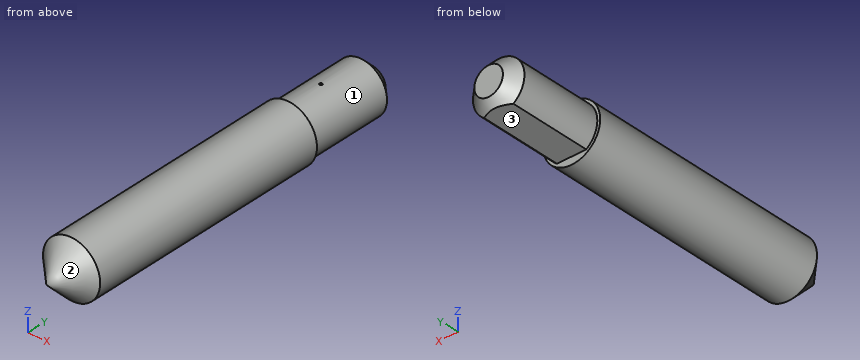
```python
from build123d import *

# Parameters (mm, degrees)
SKETCH1_R           = 5
BOSS_EXTRUDE1_DEPTH = 48
CHAMFER1_SIZE       = 5
BOSS_EXTRUDE2_DEPTH = 16.45


with BuildPart() as part:
    # Sketch1 → Boss-Extrude1 (new body)
    with BuildSketch(Plane(origin=(0, 0, 0), x_dir=(1, 0, 0), z_dir=(0, 1, 0))):
        with Locations(Location((0, 0, 0), (0, 0, 270))):
            Circle(SKETCH1_R)
    extrude(amount=BOSS_EXTRUDE1_DEPTH)

    # Chamfer1
    chamfer1_edges = [part.edges().sort_by_distance(p)[0] for p in [
        (0, 0, -5),
    ]]
    chamfer(chamfer1_edges, length=CHAMFER1_SIZE)

    # Sketch2 → Boss-Extrude2 (add)
    with BuildSketch(Plane(origin=(0, 48, 0), x_dir=(1, 0, 0), z_dir=(0, 1, 0))):
        with BuildLine():
            Line((-2.561249695, 3.7), (2.561249695, 3.7))
            ThreePointArc((2.561249695, 3.7), (0, -4.5), (-2.561249695, 3.7))
        make_face()
    extrude(amount=BOSS_EXTRUDE2_DEPTH)

    # Chamfer2: read off the stored shape, not the designer's step
    # Chamfer2 outline → Chamfer2 (revolve, cut)
    with BuildSketch(Plane.XY):
        Polygon((4.5, 64.45), (2.5, 64.45), (4.5, 62.45), align=None)
    revolve(axis=Axis((0, 0, 0), (0, 1, 0)), mode=Mode.SUBTRACT)

    # Sketch3 → Cut-Revolve1 (revolve, cut)
    with BuildSketch(Plane(origin=(0, 0, 0), x_dir=(0, 0, -1), z_dir=(1, 0, 0))):
        with BuildLine():
            Line((-4.5, 54.2), (-4.5, 54.7))
            ThreePointArc((-4.5, 54.7), (-4.25, 54.45), (-4.5, 54.2))
        make_face()
    revolve(axis=Axis((0, 54.2, 4.5), (0, 1, 0)), mode=Mode.SUBTRACT)


solid = part.part
```
Model file for the job. Use its own axes, mm. Face numbers are marked on the shaded views. A direction names the side the tool comes from. Coordinates: 2 decimals unless noted, no trailing zeros. Loops run counter-clockwise (first coordinate to the right, second up) from the corner with the lowest first, then second, coordinate; pieces in that order, holes last. Notation, with made-up numbers: (7.25, 39.25) - (61.25, 39.25) arc R29 ccw to (61.25, 59.25) - close; hole circle Ø6 at (59.5, 12.5). An arc over 180 degrees is marked (long way). Answer as a JSON object with one key per item and string values. Group by question number.
(1) Flat gauge pins, fed straight in: pin 1 (2 mm diameter, centred on x = -2.5, z = -3.5, fed in from +Y); pin 2 (1.5 mm diameter, centred on y = 39.5, z = -2, fed in from -X); pin 3 (1.5 mm diameter, centred on y = 11, z = 1, fed in from -X). Where does each tip first touch, or does it go through?
(2) Cut at A-A (y = 34). Give the cut face in (x, z), then the cut area to 3 significant figures.
(3) Probe line 1 along Y through (x, z) = (0.25, 0); line 2 along Y through (x, z) = (-2.25, -2.25); line 3 along X through (y, z) = (55.5, -1.5). List the from-to ranges inside material, lowest first.
(4) Tool access for the marked faces 1, 2 and 3: list every direction of +Z, -Z, +X, -X, +Y, -Y with a clear straight run to the whole face (end or side of a thin tool).
Geometry says:
{
 "1": {"pin 1": "stops at y = 63.65", "pin 2": "stops at x = -4.84", "pin 3": "stops at x = -4.99"},
 "2": {"outline": "circle Ø10 at (0, 0)", "area": "78.5 mm^2"},
 "3": {"line 1": "y = 0.25 to 64.45", "line 2": "y = 3.18 to 63.77", "line 3": "x = -4.24 to 4.24"},
 "4": {"face 1": "+Y", "face 2": "-Y", "face 3": "-Z, +X, -X, +Y"}
}
